The listing builds one solid part. Answer for the finished solid, in the listing's coordinates (mm). A direction names the side the tool comes from. Give positions to 0.01 mm unless a question says otherwise; leave off trailing zeros. Write each loop counter-clockwise with the first axis right and the second up, starting at its lowest first coordinate (ties: lowest second). Pieces come first, ordered by that corner, then holes. Notation, with made-up numbers: (87.25, 33.5) - (114.25, 33.5) arc R14 ccw to (114.25, 57.5) - close; hole circle Ø10 at (48, 25.25). An arc over 180 degrees is marked (long way). One line per question, with ' | ' between items. Start each with the question number.
1. Given P1, Ø7, axis at x = 25, z = -12.5, coming from the +Y side; P2, Ø13.5, axis at x = 25, z = -12.5, coming from the +Y side, each flat-ended and moving along its own axis, determine where each tip first touches the part or whether it passes through.
2. For faces 5 (the face through (31, 4, -15)), 6 (the face through (26.802, 2.028, -6.777)), determine the directions among +Z, -Z, +X, -X, +Y, -Y from which every point of the face is accessible in a straight line to the end or side of a thin tool.
3. The mould has two halves that part along Z. Classify faces 1 (the face through (1, 3, -23)), 2 (the face through (19, 0, -10)), 3 (the face through (25, 2, 0)), 4 (the face through (16.897, 4.507, -14.299)): +Z half, -Z half, draft (parallel to the pull), parting line (faces both ways), or undercut.
4. A cutting plane is placed at D-D (z = -12.75). Determine the outline of the cut face in (x, y).
5. Find the intervals of material crossed by L1, parallel to X at y = 3.15, z = -12.5; L2, parallel to X at y = 4.7, z = -12.5; L3, parallel to Y at x = 19, z = -8.25, in increasing order. Write a range as from..to.
6. A cutting plane is placed at A-A (x = 10). Determine the outline of the cut face in (y, z), then the cut area to 4 significant figures.
7. A cutting plane is placed at C-C (y = 2.45). Determine the outline of the cut face in (x, z), then the cut area to 3 significant figures.
8. A cutting plane is placed at B-B (z = -7). Determine the outline of the cut face in (x, y).
```python
from build123d import *

# Parameters (mm, degrees)
SKETCH_1_W          = 50
SKETCH_1_H          = 25
EXTRUDE_1_DEPTH     = 5
SKETCH_2_R          = 6
SKETCH_2_R_2        = 1.65
CUT_EXTRUDE_1_DEPTH = 5
SKETCH_4_R          = 8.3
CUT_EXTRUDE_2_DEPTH = 1
FILLET_1_R          = 5


with BuildPart() as part:
    # 草图1 → 凸台-拉伸1 (new body)
    with BuildSketch(Plane(origin=(0, 0, 0), x_dir=(1, 0, 0), z_dir=(0, 1, 0))):
        with Locations((25, 12.5)):
            Rectangle(SKETCH_1_W, SKETCH_1_H)
    extrude(amount=EXTRUDE_1_DEPTH)

    # 草图2 → 切除-拉伸1 (cut)
    with BuildSketch(Plane(origin=(0, 5, 0), x_dir=(1, 0, 0), z_dir=(0, 1, 0))):
        with Locations(Location((25, 12.5, 0), (0, 0, 270))):
            Circle(SKETCH_2_R)
        with Locations(Location((40, 12.5, 0), (0, 0, 270))):
            Circle(SKETCH_2_R_2)
        with Locations(Location((10, 12.5, 0), (0, 0, 270))):
            Circle(SKETCH_2_R_2)
    extrude(amount=-CUT_EXTRUDE_1_DEPTH, mode=Mode.SUBTRACT)

    # 草图4 → 切除-拉伸2 (cut)
    with BuildSketch(Plane(origin=(0, 5, 0), x_dir=(1, 0, 0), z_dir=(0, 1, 0))):
        with Locations(Location((25, 12.5, 0), (0, 0, 270))):
            Circle(SKETCH_4_R)
    extrude(amount=-CUT_EXTRUDE_2_DEPTH, mode=Mode.SUBTRACT)

    # 圆角1
    fillet_1_edges = [part.edges().sort_by_distance(p)[0] for p in [
        (0, 2.5, -25),
        (50, 2.5, -25),
        (50, 2.5, 0),
        (0, 2.5, 0),
    ]]
    fillet(fillet_1_edges, radius=FILLET_1_R)


solid = part.part
```
Determined:
1) P1: through | P2: y = 4
2) face 5: +Y | face 6: +Y, -Y
3) face 1: -Z half | face 2: draft | face 3: +Z half | face 4: undercut
4) outline: (0, 0) - (8.37, 0) - (8.37, 5) - (0, 5) - close; (11.63, 0) - (19.01, 0) - (19.01, 4) - (16.7, 4) - (16.7, 5) - (11.63, 5) - close; (30.99, 0) - (38.37, 0) - (38.37, 5) - (33.3, 5) - (33.3, 4) - (30.99, 4) - close; (41.63, 0) - (50, 0) - (50, 5) - (41.63, 5) - close
5) L1: 0..8.35, 11.65..19, 31..38.35, 41.65..50 | L2: 0..8.35, 11.65..16.7, 33.3..38.35, 41.65..50 | L3: 0..4
6) outline: (0, -25) - (5, -25) - (5, -14.15) - (0, -14.15) - close; (0, -10.85) - (5, -10.85) - (5, 0) - (0, 0) - close | area: 108.5 mm2
7) outline: (0, -20) arc R5 ccw to (5, -25) - (45, -25) arc R5 ccw to (50, -20) - (50, -5) arc R5 ccw to (45, 0) - (5, 0) arc R5 ccw to (0, -5) - close; hole circle Ø3.3 at (10, -12.5); hole circle Ø12 at (25, -12.5); hole circle Ø3.3 at (40, -12.5) | area: 1,100 mm2
8) outline: (0, 0) - (22.6, 0) - (22.6, 4) - (18.78, 4) - (18.78, 5) - (0, 5) - close; (27.4, 0) - (50, 0) - (50, 5) - (31.22, 5) - (31.22, 4) - (27.4, 4) - close
